The listing builds one solid part. Answer for the finished solid, in the listing's coordinates (mm). A direction names the side the tool comes from. Round coordinates to 2 decimals unless told otherwise and drop trailing zeros. Loops run counter-clockwise (first coordinate to the right, second up) from the corner with the lowest first, then second, coordinate; pieces in that order, holes last. Notation, with made-up numbers: (30.5, 53.25) - (62.5, 53.25) arc R11 cw to (62.5, 72.25) - close; hole circle Ø10 at (15, -2). An arc over 180 degrees is marked (long way). One line per item, written item: value.
Autodesk Inventor part; units mm, degrees
ref_plane "YZ Plane" through (0, 0, 0) normal (1, 0, 0) x (0, 1, 0)
ref_plane "XZ Plane" through (0, 0, 0) normal (0, 1, 0) x (-1, 0, 0)
ref_plane "XY Plane" through (0, 0, 0) normal (0, 0, 1) x (1, 0, 0)
sketch "Skizze1" plane through (0, 0, 0) normal (0, 0, 1) x (1, 0, 0)
  line L0 (1, 0) -> (1, 17.2649)
  line L1 (1, 17.2649) -> (2.1, 17.9)
  line L2 (2.1, 17.9) -> (2.1, 22.1)
  line L3 (2.1, 22.1) -> (3.2, 22.1)
  line L4 (3.2, 22.1) -> (3.2, 17.9)
  line L5 (3.2, 17.9) -> (3.5, 17.9)
  line L6 (3.5, 17.9) -> (3.5, 7.1)
  line L7 (3.5, 7.1) -> (1.485, 7.1)
  line L8 (1.485, 7.1) -> (1.485, 5)
  line L9 (1.485, 5) -> (3, 5)
  line L10 (3, 5) -> (3, 0)
  line L11 (3, 0) -> (1, 0)
  line L12 (0, -4.42) -> (0, 26.52)
  point P0 (0, 0)
  dimension "d0" = 120
  dimension "d1" = 1
  dimension "d2" = 1.485
  dimension "d3" = 0
  dimension "d4" = 5
  dimension "d5" = 2.1
  dimension "d6" = 15
  dimension "d7" = 2.1
  dimension "d8" = 3.5
  dimension "d9" = 3
  dimension "d10" = 0
  dimension "d11" = 4.2
  dimension "d12" = 3.2
revolve "Umdrehung1" add sketch "Skizze1" angle 360 about axis through (0, -10, 0) along (0, 1, 0)
chamfer "Fase1" distance 0.25 angle 45 2 edges at (-3.2, 22.1, 0) (-3, 0, 0)
thread "Gewinde1"
thread "Gewinde2"
properties part number "E3D-v6 1.75mm Heat Break" material "Edelstahl, 440C"
1) For faces 1 (the cylindrical face through (-2.539, 19.847, -1.947)), 2 (the cylindrical face through (-3, 3, 0)), 3 (the cylindrical face through (-0.32, 6.04, -1.45)), 4 (the flat face through (1.3, 22.1, 1.9)), determine the directions among +Z, -Z, +X, -X, +Y, -Y from which every point of the face is accessible in a straight line to the end or side of a thin tool.
Final values:
face 1: +Y
face 2: -Y
face 3: none
face 4: +Z, -Z, +X, -X, +Y
2) A cutting plane is placed at D-D on y = 14. Give the vertices of the cut face in (x, z), and give its area (3 significant figures).
Final values:
outline: circle Ø7 at (0, 0); hole circle Ø2 at (0, 0)
area: 35.3 mm2
3) A cutting plane is placed at A-A on x = 0. Give the vertices of the cut face in (y, z) (3 decimals), and give its area (3 significant figures).
Final values:
outline: (0, -2.75) - (0.25, -3) - (5, -3) - (5, -1.485) - (7.1, -1.485) - (7.1, -3.5) - (17.9, -3.5) - (17.9, -3.2) - (21.85, -3.2) - (22.1, -2.95) - (22.1, -2.1) - (17.9, -2.1) - (17.265, -1) - (0, -1) - close; (0, 1) - (17.265, 1) - (17.9, 2.1) - (22.1, 2.1) - (22.1, 2.95) - (21.85, 3.2) - (17.9, 3.2) - (17.9, 3.5) - (7.1, 3.5) - (7.1, 1.485) - (5, 1.485) - (5, 3) - (0.25, 3) - (0, 2.75) - close
area: 84.5 mm2
4) A cutting plane is placed at B-B on z = 0. Give the vertices of the cut face in (x, y) (3 decimals).
Final values:
outline: (-3.5, 7.1) - (-1.485, 7.1) - (-1.485, 5) - (-3, 5) - (-3, 0.25) - (-2.75, 0) - (-1, 0) - (-1, 17.265) - (-2.1, 17.9) - (-2.1, 22.1) - (-2.95, 22.1) - (-3.2, 21.85) - (-3.2, 17.9) - (-3.5, 17.9) - close; (1, 0) - (2.75, 0) - (3, 0.25) - (3, 5) - (1.485, 5) - (1.485, 7.1) - (3.5, 7.1) - (3.5, 17.9) - (3.2, 17.9) - (3.2, 21.85) - (2.95, 22.1) - (2.1, 22.1) - (2.1, 17.9) - (1, 17.265) - close
5) This flat-tipped pin is pushed along its axis until it touches: pin 1 Ø4 at (x, y) = (-2.5, 7.5) entering from +Z. Where does it stop, or does it pass through?
Final values:
pin 1: z = 3.46
6) For a pull along Z with two mould halves and no side action, classify faces 5 (the flat face through (1.3, 5, 1.3)), 6 (the cylindrical face through (3.233, 12.424, -1.341)), 7 (the cylindrical face through (0, 9, 1)) as released by +Z, released by -Z, zero draft, split by the parting line, or undercut.
Final values:
face 5: zero draft
face 6: split by the parting line
face 7: undercut
7) Consider L1, parallel to X at y = 20, z = 0; L2, parallel to X at y = 9, z = 0. Determine where each line is inside the solid, lowest interval first.
Final values:
L1: -3.2 to -2.1, 2.1 to 3.2
L2: -3.5 to -1, 1 to 3.5
8) A cutting plane is placed at C-C on y = 19.75. Give the vertices of the cut face in (x, z).
Final values:
outline: circle Ø6.4 at (0, 0); hole circle Ø4.2 at (0, 0)
